from build123d import *

# Parameters (mm, degrees)
SKIZZE1_R                       = 1.7
AUFSATZ_LINEAR_AUSTRAGEN1_DEPTH = 0.8
AUFSATZ_LINEAR_AUSTRAGEN2_DEPTH = 1


with BuildPart() as part:
    # Skizze1 → Aufsatz-Linear austragen1 (new body)
    with BuildSketch(Plane.XY):
        with BuildLine():
            Line((0, 5), (0, 82.7))
            ThreePointArc((0, 82.7), (1.464466094, 86.235533906), (5, 87.7))
            Line((5, 87.7), (21.9, 87.7))
            Line((21.9, 87.7), (21.9, 79.73388451))
            Line((21.9, 79.73388451), (55.9, 79.73388451))
            Line((55.9, 79.73388451), (55.9, 87.7))
            Line((55.9, 87.7), (114.2, 87.7))
            ThreePointArc((114.2, 87.7), (117.735533906, 86.235533906), (119.2, 82.7))
            Line((119.2, 82.7), (119.2, 75.8))
            Line((119.2, 75.8), (119.2, 5))
            ThreePointArc((119.2, 5), (117.735533906, 1.464466094), (114.2, 0))
            Line((114.2, 0), (5, 0))
            ThreePointArc((5, 0), (1.464466094, 1.464466094), (0, 5))
        make_face()
        with Locations((3.2, 9.6)):
            Circle(SKIZZE1_R, mode=Mode.SUBTRACT)
        with Locations((3.2, 78.1)):
            Circle(SKIZZE1_R, mode=Mode.SUBTRACT)
        with Locations((114.35, 82.85)):
            Circle(SKIZZE1_R, mode=Mode.SUBTRACT)
        with Locations((114.35, 4.85)):
            Circle(SKIZZE1_R, mode=Mode.SUBTRACT)
    extrude(amount=AUFSATZ_LINEAR_AUSTRAGEN1_DEPTH)

    # Skizze3 → Aufsatz-Linear austragen2 (add)
    with BuildSketch(Plane(origin=(0, 0, 0), x_dir=(-1, 0, 0), z_dir=(0, 0, -1))):
        Polygon((-55.9, 79.73388451), (-55.9, 85.1), (-105.458578644, 85.1), (-117.5, 73.058578644), (-117.5, 14.641421356), (-105.458578644, 2.6), (-6.5, 2.6), (-6.5, 17.286335909), (-1.7, 22.086335909), (-1.7, 66.058578644), (-6.5, 70.858578644), (-6.5, 85.1), (-21.9, 85.1), (-21.9, 79.73388451), align=None)
        Polygon((-58.844037441, 83.9), (-57.1, 83.9), (-57.1, 78.53388451), (-20.7, 78.53388451), (-20.7, 83.9), (-7.7, 83.9), (-7.7, 82.43185957), (-58.844037441, 45.143695389), align=None, mode=Mode.SUBTRACT)
        Polygon((-104.961522369, 83.9), (-60.044037441, 83.9), (-60.044037441, 45.139977904), (-108.547677312, 80.313845057), align=None, mode=Mode.SUBTRACT)
        Polygon((-116.3, 72.561522369), (-109.406904246, 79.454618123), (-61.293455008, 44.563709394), (-116.3, 44.563709394), align=None, mode=Mode.SUBTRACT)
        Polygon((-116.3, 15.138477631), (-116.3, 43.363709394), (-61.293455008, 43.363709394), (-109.538727473, 8.377205104), align=None, mode=Mode.SUBTRACT)
        Polygon((-104.961522369, 3.8), (-108.679500539, 7.51797817), (-60.044037441, 42.787440884), (-60.044037441, 3.8), align=None, mode=Mode.SUBTRACT)
        Polygon((-7.5, 3.8), (-58.844037441, 3.8), (-58.844037441, 42.7837234), (-7.5, 5.349742948), align=None, mode=Mode.SUBTRACT)
        Polygon((-7.5, 17.983392184), (-7.5, 6.834817309), (-57.602628153, 43.363709394), (-2.9, 43.363709394), (-2.9, 22.583392184), align=None, mode=Mode.SUBTRACT)
        Polygon((-2.9, 65.561522369), (-2.9, 44.563709394), (-57.602628153, 44.563709394), (-7.7, 80.946785208), (-7.7, 70.361522369), align=None, mode=Mode.SUBTRACT)
    extrude(amount=AUFSATZ_LINEAR_AUSTRAGEN2_DEPTH)


solid = part.part
Source: CAD feature listing. Evaluate the final solid. Frame: model axes, mm. A direction names the side the tool comes from. Coordinates: 2 decimals unless noted, no trailing zeros. Loops run counter-clockwise (first coordinate to the right, second up) from the corner with the lowest first, then second, coordinate; pieces in that order, holes last. Notation, with made-up numbers: (-16, 20) -> (14, 20) arc R6 cw to (14, 24) -> close; hole circle Ø2 at (-37, 84.5). An arc over 180 degrees is marked (long way). Answer in a Markdown table with one row per item. Add a question column.
Q1. Ray query, line 1 along Y through (x, z) = (114.35, 0.5); line 2 along X through (y, z) = (82.85, 0.2); line 3 along X through (y, z) = (35.5, -0.5). Return the intervals inside material, ascending.
Q2. Section A-A on z = 0.5. Return the cut outline in (x, y), and give its area (3 significant figures).
Q3. Section B-B on y = 9.6. Return the cut outline in (x, z).
Q4. Pull-direction query (X, two-part tool) for faces 1 (the face through (60, 44, -1)), 2 (the face through (32.201, 24.844, -0.493)), 3 (the face through (111.564, 8.705, -0.493)); classes: pulls with the +X half, pulls with the -X half, needs draft (parallel to the pull), parting line crosses it, or undercut.
Q5. Section C-C on y = 34. Return the cut outline in (x, z), and give its area (3 significant figures).
Q6. Section D-D on x = 74. Return the cut outline in (y, z).
Q7. Reachability of faces 4 (the face through (25, 55, 0)), 5 (the face through (4.066, 68.425, -0.493)), 6 (the face through (117.7, 86.27, 0.39)) from +Z, -Z, +X, -X, +Y, -Y: full face, straight path, thin tool, end or side. Return the list, or none.
Q8. Contact query for flat-ended pins moving along their axis: pin 1 Ø0.8 at (y, z) = (80.5, -0.5) entering from -X; pin 2 Ø0.5 at (y, z) = (27, -0.5) entering from -X; pin 3 Ø0.9 at (x, z) = (38.5, 0) entering from +Y. Output: stop coordinate, or through.
Computed values:
| question | item | result |
|---|---|---|
| 1 | line 1 | y = 0 to 3.15, 6.55 to 81.15, 84.55 to 87.7 |
| 1 | line 2 | x = 0 to 21.9, 55.9 to 112.65, 116.05 to 119.2 |
| 1 | line 3 | x = 1.7 to 2.9, 46.82 to 48.85, 58.84 to 60.04, 70.09 to 72.14, 116.3 to 117.5 |
| 2 | outline | (0, 5) arc R5 ccw to (5, 0) -> (114.2, 0) arc R5 ccw to (119.2, 5) -> (119.2, 82.7) arc R5 ccw to (114.2, 87.7) -> (55.9, 87.7) -> (55.9, 79.73) -> (21.9, 79.73) -> (21.9, 87.7) -> (5, 87.7) arc R5 ccw to (0, 82.7) -> close; hole circle Ø3.4 at (3.2, 9.6); hole circle Ø3.4 at (3.2, 78.1); hole circle Ø3.4 at (114.35, 4.85); hole circle Ø3.4 at (114.35, 82.85) |
| 2 | area | 10,100 mm^2 |
| 3 | outline | (0, 0) -> (1.5, 0) -> (1.5, 0.8) -> (0, 0.8) -> close; (4.9, 0) -> (6.5, 0) -> (6.5, -1) -> (7.5, -1) -> (7.5, 0) -> (11.29, 0) -> (11.29, -1) -> (13.33, -1) -> (13.33, 0) -> (58.84, 0) -> (58.84, -1) -> (60.04, -1) -> (60.04, 0) -> (105.81, 0) -> (105.81, -1) -> (107.85, -1) -> (107.85, 0) -> (110.76, 0) -> (110.76, -1) -> (112.46, -1) -> (112.46, 0) -> (119.2, 0) -> (119.2, 0.8) -> (4.9, 0.8) -> close |
| 4 | face 1 | needs draft |
| 4 | face 2 | undercut |
| 4 | face 3 | pulls with the +X half |
| 5 | outline | (0, 0) -> (1.7, 0) -> (1.7, -1) -> (2.9, -1) -> (2.9, 0) -> (44.76, 0) -> (44.76, -1) -> (46.8, -1) -> (46.8, 0) -> (58.84, 0) -> (58.84, -1) -> (60.04, -1) -> (60.04, 0) -> (72.16, 0) -> (72.16, -1) -> (74.21, -1) -> (74.21, 0) -> (116.3, 0) -> (116.3, -1) -> (117.5, -1) -> (117.5, 0) -> (119.2, 0) -> (119.2, 0.8) -> (0, 0.8) -> close |
| 5 | area | 103 mm^2 |
| 6 | outline | (0, 0) -> (2.6, 0) -> (2.6, -1) -> (3.8, -1) -> (3.8, 0) -> (32.67, 0) -> (32.67, -1) -> (34.15, -1) -> (34.15, 0) -> (43.36, 0) -> (43.36, -1) -> (44.56, -1) -> (44.56, 0) -> (53.78, 0) -> (53.78, -1) -> (55.26, -1) -> (55.26, 0) -> (83.9, 0) -> (83.9, -1) -> (85.1, -1) -> (85.1, 0) -> (87.7, 0) -> (87.7, 0.8) -> (0, 0.8) -> close |
| 7 | face 4 | -Z |
| 7 | face 5 | -Z, -X, +Y |
| 7 | face 6 | +Z, -Z, +X, +Y |
| 8 | pin 1 | stops at x = 6.5 |
| 8 | pin 2 | stops at x = 1.7 |
| 8 | pin 3 | stops at y = 79.73 |
